```python
from build123d import *

# Parameters (mm, degrees)
EXTRUDE_1_DEPTH     = 80
EXTRUDE_4_DEPTH     = 20
HOLE_WIZARD_M5_1_D  = 4.2
HOLE_WIZARD_M6_1_D  = 5
SKETCH_2_R          = 17.5
CUT_EXTRUDE_2_DEPTH = 116.866302263


with BuildPart() as part:
    # 草图1 → 拉伸1 (new body)
    with BuildSketch(Plane.XY):
        Polygon((0, 0), (80, 0), (80, 25), (60, 25), (60, 10), (20, 10), (20, 25), (0, 25), align=None)
    extrude(amount=EXTRUDE_1_DEPTH)

    # 草图7 → 拉伸4 (add)
    with BuildSketch(Plane(origin=(0, 0, 0), x_dir=(-1, 0, 0), z_dir=(0, 0, -1))):
        Polygon((-80, 0), (-80, 25), (-60, 25), (-60, 10), (-20, 10), (-20, 25), (0, 25), (0, 0), align=None)
    extrude(amount=EXTRUDE_4_DEPTH)

    # M5 螺纹孔1 (through all)
    with Locations(Plane(origin=(73.234018716, 0, 72.779084328), x_dir=(0, 0, -1), z_dir=(0, -1, 0))):
        with Locations((0, 0), (0, -66.468037432), (66.468037432, -66.468037432), (66.468037432, 0)):
            Hole(HOLE_WIZARD_M5_1_D / 2)

    # M6 螺纹孔1 (through all)
    with Locations(Plane(origin=(0, 25, 0), x_dir=(-1, 0, 0), z_dir=(0, 1, 0))):
        with Locations((-15, -10), (-15, 60), (-65, -10), (-65, 60)):
            Hole(HOLE_WIZARD_M6_1_D / 2)

    # 草图2 → 拉伸2 (cut, through all)
    with BuildSketch(Plane(origin=(0, 0, 0), x_dir=(1, 0, 0), z_dir=(0, 1, 0))):
        with Locations(Location((40, -24.55, 0), (0, 0, 90))):
            Circle(SKETCH_2_R)
    extrude(amount=CUT_EXTRUDE_2_DEPTH, mode=Mode.SUBTRACT)


solid = part.part
```
The model under review builds one solid part; all positions refer to its coordinate system, in mm. A direction names the side the tool comes from. Round coordinates to 2 decimals unless told otherwise and drop trailing zeros. Write each loop counter-clockwise with the first axis right and the second up, starting at its lowest first coordinate (ties: lowest second). Pieces come first, ordered by that corner, then holes. Notation, with made-up numbers: M -35,-25 L -27,-25 A18 cw -27,-16 Z; hole C -10,6.25 d10. An arc over 180 degrees is marked long. Use CSV: the item, a comma, the result in double quotes. Start each with the question number.
(1) The part is to be moulded in two halves that separate along X. For faces 1 (the face through (80, 12, 31)), 2 (the face through (70, 25, 31)), 3 (the face through (8.85, 12.68, 6.04)), say which applies: +X half, -X half, draft (parallel to the pull), parting line (faces both ways), or undercut.
(2) Clearance check with flat-ended pins moving along their axes: P1, Ø8, axis at x = 43.5, z = 36.5, coming from the +Y side; P2, Ø20, axis at x = 44, z = 36, coming from the +Y side. State where each tip first meets the part, or that it passes through.
(3) We need section B-B, the plane y = 17.5. State how many separate pieces and enclosed holes the cut face has, then the cut area to 3 significant figures.
(4) We need section A-A, the plane z = 24.55. State the section outline as (x, y) points, then the cut area to 3 significant figures.
(5) Tool access review of faces 4 (the face through (13, 12.3, -11.5)), 5 (the face through (45, 10, 42)): name each direction out of +Z, -Z, +X, -X, +Y, -Y from which nothing blocks a thin tool from reaching the whole face with its end or side.
(6) We need section C-C, the plane x = 65. State the section outline as (y, z) points, then the cut area to 3 significant figures.
(7) We need section D-D, the plane z = -10. State the section outline as (x, y) points, then the cut area to 3 significant figures.
(8) For line 1 along Z through (x, y) = (65, 18.75); line 2 along Z through (x, y) = (7, 19.75); line 3 along X through (y, z) = (20, 3), list the stretches that pass through material, from the lowest coordinate up.
Findings:
1,face 1,"+X half"
1,face 2,"draft"
1,face 3,"undercut"
2,P1,"through"
2,P2,"y = 10"
3,separate pieces,"2"
3,enclosed holes,"8"
3,area,"3,870 mm^2"
4,outline,"M 0,0 L 22.5,0 L 22.5,10 L 20,10 L 20,25 L 0,25 Z; M 57.5,0 L 80,0 L 80,25 L 60,25 L 60,10 L 57.5,10 Z"
4,area,"1,050 mm^2"
5,face 4,"+Y, -Y"
5,face 5,"+Z, -Z, +Y"
6,outline,"M 0,-20 L 25,-20 L 25,-12.5 L 0,-12.5 Z; M 0,-7.5 L 25,-7.5 L 25,57.5 L 0,57.5 Z; M 0,62.5 L 25,62.5 L 25,80 L 0,80 Z"
6,area,"2,250 mm^2"
7,outline,"M 0,0 L 12.5,0 L 12.5,25 L 0,25 Z; M 17.5,0 L 62.5,0 L 62.5,25 L 60,25 L 60,10 L 20,10 L 20,25 L 17.5,25 Z; M 67.5,0 L 80,0 L 80,25 L 67.5,25 Z"
7,area,"1,150 mm^2"
8,line 1,"-20 to -12.5, -7.5 to 57.5, 62.5 to 80"
8,line 2,"-20 to 4.22, 8.4 to 70.69, 74.87 to 80"
8,line 3,"0 to 20, 60 to 80"
